Work out the finished part from the listing and answer in its coordinate system (mm). A direction names the side the tool comes from. Round coordinates to 2 decimals unless told otherwise and drop trailing zeros. Order: outer loops, then holes, each group sorted by start corner. A loop starts at its lowest first (then second) coordinate and runs counter-clockwise, first axis right, second up. Notation, with made-up numbers: (32, 87.25) -> (44, 87.25) arc R26 cw to (44, 105.25) -> close; hole circle Ø10 at (-32.75, 58.25). An arc over 180 degrees is marked (long way). Use a Markdown table: item, result. Add a question column.
Item 1: A tool of negligible diameter and unlimited length cuts with its end or side. For faces 4 (the cylindrical face through (-11.923, 0.986, 3.755)), 5 (the flat face through (3, -8.483, -8.2)), from which of +Z, -Z, +X, -X, +Y, -Y can it reach the whole face along a straight path? Write none if from no direction.
Item 2: A cutting plane is placed at B-B, the plane x = 9. Determine the outline of the cut face in (y, z).
Item 3: Find the intervals of material crossed by L1, parallel to Z at x = 0, y = -14.5; L2, parallel to Y at x = -10.75, z = -0.25; L3, parallel to X at y = -10, z = -4, in increasing order. Write a range as [from, to].
Item 4: A cutting plane is placed at D-D, the plane z = 0. Determine the outline of the cut face in (x, y).
Item 5: Flat-ended cylindrical pins translate along their axes: P1, Ø8, axis at x = 5, y = -2.5, coming from the +Z side; P2, Ø4, axis at x = -4, z = 2, coming from the +Y side; P3, Ø2, axis at x = 7, y = 2.5, coming from the -Z side. Find the tip coordinate at first contact, or state that the pin passes through.
Item 6: For a pull along Z with two mould halves and no side action, classify faces 1 (the flat face through (0.2, 0, -5.4)), 2 (the cylindrical face through (0, 3, -2)), 3 (the cylindrical face through (-1.08, -8.53, -4.88)) as +Z half, -Z half, draft (parallel to the pull), parting line (faces both ways), or undercut.
Item 7: A cutting plane is placed at C-C, the plane y = -16. Determine the outline of the cut face in (x, z), plus the area to 3 significant figures.
Item 8: A cutting plane is placed at A-A, the plane z = 7.5. Determine the outline of the cut face in (x, y), plus the area to 3 significant figures.
from build123d import *

# Parameters (mm, degrees)
F0_R      = 5
F1_DEPTH  = 17.3
F2_R      = 12.5
F3_DEPTH  = 2
F4_R      = 12.5
F4_R_2    = 8.5
F5_DEPTH  = 8.817
F6_R      = 12.5
F7_DEPTH  = 2
F8_R      = 2
F9_DEPTH  = 5
F10_R     = 2
F11_R     = 12.5
F12_DEPTH = 5


with BuildPart() as f1:
    # F0 (on Front) → F1 (new body)
    with BuildSketch(Plane.XZ):
        Circle(F0_R)
    extrude(amount=F1_DEPTH)

    # F2 (on face) → F3 (join)
    with BuildSketch(Plane.XZ.offset(17.3)):
        Circle(F2_R)
    extrude(amount=F3_DEPTH)

    # F4 (on face) → F5 (join)
    with BuildSketch(Plane(origin=(0, -17.3, 0), x_dir=(-1, 0, 0), z_dir=(0, 1, 0))):
        Circle(F4_R)
        Circle(F4_R_2, mode=Mode.SUBTRACT)
    extrude(amount=F5_DEPTH)

    # F6 (on face) → F7 (join)
    with BuildSketch(Plane(origin=(0, 0, 0), x_dir=(-1, 0, 0), z_dir=(0, 1, 0))):
        Circle(F6_R)
    extrude(amount=F7_DEPTH)

    # F8 (on face) → F9 (join)
    with BuildSketch(Plane(origin=(0, 2, 0), x_dir=(-1, 0, 0), z_dir=(0, 1, 0))):
        Circle(F8_R)
    extrude(amount=F9_DEPTH)

    # F10
    f10_edges = [f1.edges().sort_by_distance(p)[0] for p in [
        (2, 7, 0),
    ]]
    fillet(f10_edges, radius=F10_R)

    # F11 (on face) → F12 (join)
    with BuildSketch(Plane.XZ.offset(19.3)):
        Circle(F11_R)
    extrude(amount=F12_DEPTH)


solid = f1.part
Reported:
| question | item | result |
|---|---|---|
| 1 | face 4 | +Y, -Y |
| 1 | face 5 | none |
| 2 | outline | (-24.3, -8.67) -> (-8.48, -8.67) -> (-8.48, 8.67) -> (-24.3, 8.67) -> close; (0, -8.67) -> (2, -8.67) -> (2, 8.67) -> (0, 8.67) -> close |
| 3 | L1 | [-12.5, -8.5], [-5, 5], [8.5, 12.5] |
| 3 | L2 | [-24.3, -8.48], [0, 2] |
| 3 | L3 | [-11.84, -7.5], [-3, 3], [7.5, 11.84] |
| 4 | outline | (-12.5, -24.3) -> (12.5, -24.3) -> (12.5, -8.48) -> (8.5, -8.48) -> (8.5, -17.3) -> (5, -17.3) -> (5, 0) -> (12.5, 0) -> (12.5, 2) -> (2, 2) -> (2, 5) arc R2 ccw to (-2, 5) -> (-2, 2) -> (-12.5, 2) -> (-12.5, 0) -> (-5, 0) -> (-5, -17.3) -> (-8.5, -17.3) -> (-8.5, -8.48) -> (-12.5, -8.48) -> close |
| 5 | P1 | z = 12.36 |
| 5 | P2 | y = 2 |
| 5 | P3 | z = -10.89 |
| 6 | face 1 | draft |
| 6 | face 2 | parting line |
| 6 | face 3 | undercut |
| 7 | outline | circle Ø25 at (0, 0); circle Ø10 at (0, 0); hole circle Ø17 at (0, 0) |
| 7 | area | 342 mm² |
| 8 | outline | (-10, -24.3) -> (10, -24.3) -> (10, -8.48) -> (4, -8.48) -> (4, -17.3) -> (-4, -17.3) -> (-4, -8.48) -> (-10, -8.48) -> close; (-10, 0) -> (10, 0) -> (10, 2) -> (-10, 2) -> close |
| 8 | area | 286 mm² |
